from build123d import *

# Parameters (mm, degrees)
BOSS_EXTRUDE1_DEPTH     = 4
CUT_EXTRUDE1_DEPTH      = 14.124404748
CUT_EXTRUDE1_DEPTH_BACK = 14.124404748
SKETCH2_R               = 2
CUT_EXTRUDE2_DEPTH      = 14.124404748
CUT_EXTRUDE2_DEPTH_BACK = 14.124404748
CUT_EXTRUDE3_DEPTH      = 10.861541462
CUT_EXTRUDE3_DEPTH_BACK = 10.861541462
CUT_EXTRUDE4_DEPTH      = 16.394804318
CUT_EXTRUDE4_DEPTH_BACK = 16.394804318
SKETCH8_R               = 2


with BuildPart() as part:
    # Sketch1 → Boss-Extrude1 (new, symmetric)
    with BuildSketch(Plane(origin=(0, 0, 0), x_dir=(0, 0, -1), z_dir=(1, 0, 0))):
        Polygon((2.5, 7.5), (5, 7.5), (5, -2.5), (3, -7.5), (-3, -7.5), (-5, -2.5), (-5, 7.5), (-2.5, 7.5), (-2.5, -2.5), (2.5, -2.5), align=None)
    extrude(amount=BOSS_EXTRUDE1_DEPTH, both=True)

    # Sketch2 → Cut-Extrude1 (cut, two sides: drawn at the far end of the back side and taken through both)
    with BuildSketch(Plane.XY.offset(5).offset(-CUT_EXTRUDE1_DEPTH_BACK)):
        with Locations((0, 2.5)):
            Circle(SKETCH2_R)
    extrude(amount=CUT_EXTRUDE1_DEPTH + CUT_EXTRUDE1_DEPTH_BACK, mode=Mode.SUBTRACT)

    # Sketch3 → Cut-Extrude2 (cut, two sides: drawn at the far end of the back side and taken through both)
    with BuildSketch(Plane.XY.offset(5).offset(-CUT_EXTRUDE2_DEPTH_BACK)):
        with BuildLine():
            Line((-4, 2.5), (-4, 7.5))
            Line((-4, 7.5), (4, 7.5))
            Line((4, 7.5), (4, 2.5))
            ThreePointArc((4, 2.5), (0, 6.5), (-4, 2.5))
        make_face()
    extrude(amount=CUT_EXTRUDE2_DEPTH + CUT_EXTRUDE2_DEPTH_BACK, mode=Mode.SUBTRACT)

    # Sketch5 → Cut-Extrude3 (cut, two sides: drawn at the far end of the back side and taken through both)
    with BuildSketch(Plane.XY.offset(-CUT_EXTRUDE3_DEPTH_BACK)):
        Polygon((-4, -2.5), (-4, -7.5), (-3, -7.5), align=None)
        Polygon((3, -7.5), (4, -2.5), (4, -7.5), align=None)
    extrude(amount=CUT_EXTRUDE3_DEPTH + CUT_EXTRUDE3_DEPTH_BACK, mode=Mode.SUBTRACT)

    # Sketch8 → Cut-Extrude4 (cut, two sides: drawn at the far end of the back side and taken through both)
    with BuildSketch(Plane.XZ.offset(7.5).offset(-CUT_EXTRUDE4_DEPTH_BACK)):
        with Locations(Location((0, 0, 0), (0, 0, 270))):
            Circle(SKETCH8_R)
    extrude(amount=CUT_EXTRUDE4_DEPTH + CUT_EXTRUDE4_DEPTH_BACK, mode=Mode.SUBTRACT)


solid = part.part
Can you work these out from the model? Positions are in its coordinate system, mm. A direction names the side the tool comes from. Give positions to 0.01 mm unless a question says otherwise; leave off trailing zeros. Loops run counter-clockwise (first coordinate to the right, second up) from the corner with the lowest first, then second, coordinate; pieces in that order, holes last. Notation, with made-up numbers: M -30.75,-6 L -12.75,-6 A17 ccw -12.75,1 Z; hole C 37,24.25 d3. An arc over 180 degrees is marked long. One line per item, written item: value. Start each with the question number.
1) If we section it at D-D, the plane z = 2.75: Write out the boundary of the cut face in (x, y).
2) If we section it at A-A, the plane y = 0: Write out the boundary of the cut face in (x, z).
3) If we section it at B-B, the plane x = 0: Write out the boundary of the cut face in (y, z).
4) I'm going to push flat-ended pins straight in: pin 1 (1.5 mm diameter, centred on y = 3, z = -1.5, fed in from +X); pin 2 (1 mm diameter, centred on y = -4, z = 0, fed in from -X); pin 3 (1 mm diameter, centred on y = -5.5, z = -2, fed in from +X). Where does each tip first touch, or does it pass through?
5) Thinking about a two-plate mould opening in Y: for faces 3 (the face through (-4, 0, -4)), 4 (the face through (-0.434, 0.548, 3.732)), 5 (the face through (0.1, 6.5, -3.8)), which applies, +Y half, -Y half, draft (parallel to the pull), parting line (faces both ways), or undercut?
6) If we section it at C-C, the plane z = 0: Write out the boundary of the cut face in (x, y).
7) On a 3-axis mill with a long thin cutter (end or side, diameter ignored), from which of +Z, -Z, +X, -X, +Y, -Y can I reach the whole of each face in a straight line? I mean faces 1 (the face through (0, 0, 2.5)), 2 (the face through (4, 0, -4)). Say none if no direction works.
8) If I drill on line 1 (X direction, y = 2.5, z = 3.15); line 2 (Z direction, x = 2, y = -0.75), over which ranges is the centre line in solid material (lowest first)? Write a range as [from, to].
Completed:
1. outline: M -4,-2.5 L -3,-7.5 L 3,-7.5 L 4,-2.5 L 4,2.5 A4 ccw -4,2.5 Z; hole C 0,2.5 d4
2. outline: M -4,-5 L 4,-5 L 4,-2.5 L -4,-2.5 Z; M -4,2.5 L 4,2.5 L 4,5 L -4,5 Z
3. outline: M -7.5,-3 L -2.5,-5 L 0.5,-5 L 0.5,-2.5 L -2.5,-2.5 L -2.5,-2 L -7.5,-2 Z; M -7.5,2 L -2.5,2 L -2.5,2.5 L 0.5,2.5 L 0.5,5 L -2.5,5 L -7.5,3 Z; M 4.5,-5 L 6.5,-5 L 6.5,-2.5 L 4.5,-2.5 Z; M 4.5,2.5 L 6.5,2.5 L 6.5,5 L 4.5,5 Z
4. pin 1: passes through
4. pin 2: stops at x = -3.8
4. pin 3: stops at x = 3.5
5. face 3: draft
5. face 4: undercut
5. face 5: +Y half
6. outline: M -4,-2.5 L -3,-7.5 L -2,-7.5 L -2,-2.5 Z; M 2,-7.5 L 3,-7.5 L 4,-2.5 L 2,-2.5 Z
7. face 1: +X, -X, +Y
7. face 2: +Z, -Z, +X, +Y, -Y
8. line 1: x = [-4, -2], [2, 4]
8. line 2: z = [-5, -2.5], [2.5, 5]
